```python
from build123d import *

# Parameters (mm, degrees)
ESBO_O1_W                = 27.5
ESBO_O1_H                = 30
RESSALTO_EXTRUS_O1_DEPTH = 6


with BuildPart() as part:
    # Esboço1 → Ressalto-extrusão1 (new body)
    with BuildSketch(Plane.XY):
        Polygon((75, 75), (75, 0), (105, 0), (105, 75), (105, 105), (105, 180), (90, 180), (75, 180), (75, 105), (0, 105), (0, 75), align=None)
        with Locations((118.75, 90)):
            Rectangle(ESBO_O1_W, ESBO_O1_H)
    extrude(amount=RESSALTO_EXTRUS_O1_DEPTH)


solid = part.part
```
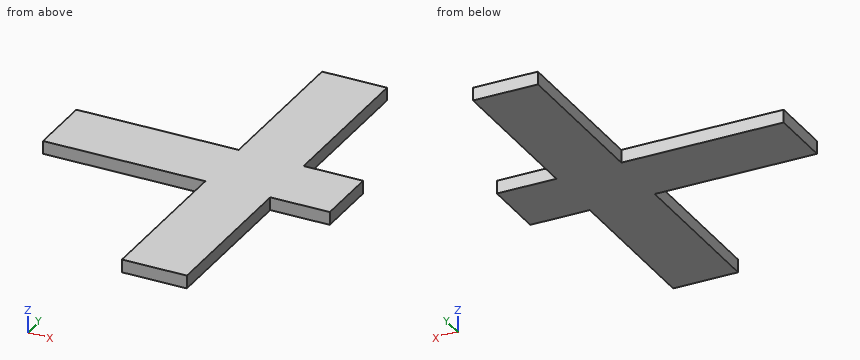
Work out the finished part from the listing and answer in its coordinate system (mm). Round coordinates to 2 decimals unless told otherwise and drop trailing zeros. Loops run counter-clockwise (first coordinate to the right, second up) from the corner with the lowest first, then second, coordinate; pieces in that order, holes last.
(1) The part is cut by section B-B, the plane x = 116.5. Give the vertices of the cut face in (y, z).
Computed values:
outline: (75, 0) - (105, 0) - (105, 6) - (75, 6) - close
(2) Find the intervals of material crossed by L1, parallel to Y at x = 36.5, z = 3.1, in increasing order.
Computed values:
L1: y = 75 to 105
(3) Each of these flat-tipped pins is pushed along its axis until it touches: P1, Ø1.8, axis at x = 112.5, z = 3.5, coming from the -Y side; P2, Ø3, axis at y = 107.5, z = 2.5, coming from the -X side; P3, Ø1.8, axis at y = 129.5, z = 3.5, coming from the +X side. Where does it stop, or does it pass through?
Computed values:
P1: stops at y = 75
P2: stops at x = 75
P3: stops at x = 105
(4) The part is cut by section A-A, the plane z = 4.05. Give the vertices of the cut face in (x, y).
Computed values:
outline: (0, 75) - (75, 75) - (75, 0) - (105, 0) - (105, 75) - (132.5, 75) - (132.5, 105) - (105, 105) - (105, 180) - (75, 180) - (75, 105) - (0, 105) - close
